Could you check a few things on this drawing? It's one solid part, dimensions in mm from its lowest x, y, z. A direction names the side the tool comes from. Give positions to 0.01 mm unless a question says otherwise; leave off trailing zeros. Write each loop counter-clockwise with the first axis right and the second up, starting at its lowest first coordinate (ties: lowest second). Pieces come first, ordered by that corner, then holes.
1. If I drill on probe 1 along Z at (x, y) = (5, 6.25); probe 2 along Y at (x, z) = (34, 25); probe 3 along X at (y, z) = (3, 3.5), over which ranges is the centre line in solid material (lowest first)?
2. Suppose I cut it at D-D (y = 11.5). Please give me the cut outline in (x, z).
3. I'm going to push flat-ended pins straight in: pin 1 (4 mm diameter, centred on x = 26.5, z = 42.5, fed in from -Y); pin 2 (1 mm diameter, centred on x = 15.5, y = 9.5, fed in from +Z); pin 3 (3 mm diameter, centred on x = 16.5, y = 5.5, fed in from -Z); pin 4 (5 mm diameter, centred on y = 4, z = 35.5, fed in from +X). Where does each tip first touch, or does it pass through?
4. Suppose I cut it at B-B (x = 34.5). Please give me the cut outline in (y, z).
5. Suppose I cut it at C-C (z = 20). Please give me the cut outline in (x, y).
6. On a 3-axis mill with a long thin cutter (end or side, diameter ignored), from which of +Z, -Z, +X, -X, +Y, -Y can I reach the whole of each face in a straight line? I mean the marked faces 1, 2, 3, 4 and 5. Say none if no direction works.
7. Suppose I cut it at A-A (y = 6.35). Please give me the cut outline in (x, z), and give its area (3 significant figures).
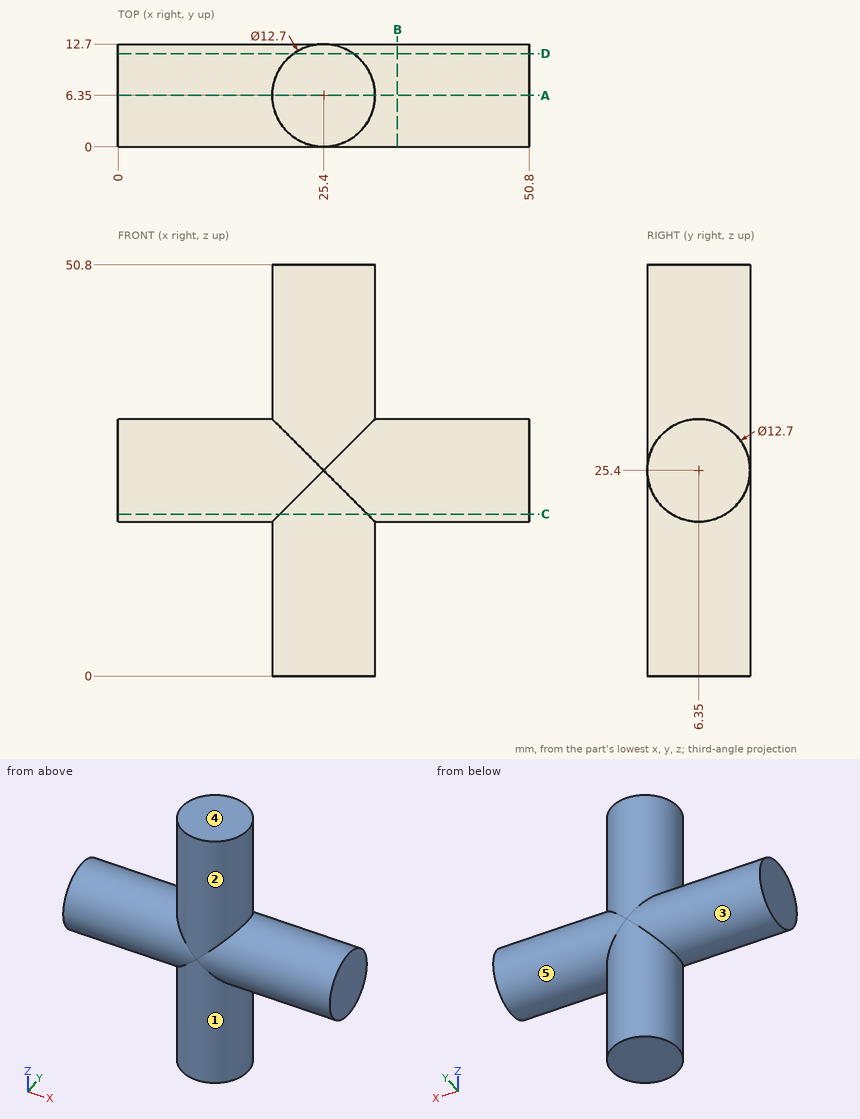
Checks:
1. probe 1: z = 19.05 to 31.75
1. probe 2: y = 0.01 to 12.69
1. probe 3: x = 20.01 to 30.79
2. outline: (0, 21.69) - (21.69, 21.69) - (21.69, 0) - (29.11, 0) - (29.11, 21.69) - (50.8, 21.69) - (50.8, 29.11) - (29.11, 29.11) - (29.11, 50.8) - (21.69, 50.8) - (21.69, 29.11) - (0, 29.11) - close
3. pin 1: stops at y = 0
3. pin 2: stops at z = 31.17
3. pin 3: stops at z = 19.05
3. pin 4: stops at x = 31.75
4. outline: circle Ø12.7 at (6.35, 25.4)
5. outline: (0, 3.01) - (20, 3.01) arc R6.35 ccw to (30.8, 3.01) - (50.8, 3.01) - (50.8, 9.69) - (30.8, 9.69) arc R6.35 ccw to (20, 9.69) - (0, 9.69) - close
6. face 1: -Z
6. face 2: +Z
6. face 3: -X
6. face 4: +Z, +X, -X, +Y, -Y
6. face 5: +X
7. outline: (0, 19.05) - (19.05, 19.05) - (19.05, 0) - (31.75, 0) - (31.75, 19.05) - (50.8, 19.05) - (50.8, 31.75) - (31.75, 31.75) - (31.75, 50.8) - (19.05, 50.8) - (19.05, 31.75) - (0, 31.75) - close
7. area: 1,130 mm2
